Check sheet for the modelled part. Datum: model origin and axes. Units: mm. Coordinates: 2 decimals unless noted, no trailing zeros. Write each loop counter-clockwise with the first axis right and the second up, starting at its lowest first coordinate (ties: lowest second). Pieces come first, ordered by that corner, then holes. Notation, with made-up numbers: (-26, -12) -> (13, -12) arc R21 ccw to (13, 26) -> close; hole circle Ø1 at (41.25, -20). An arc over 180 degrees is marked (long way). Put each result on its own line as item: value.
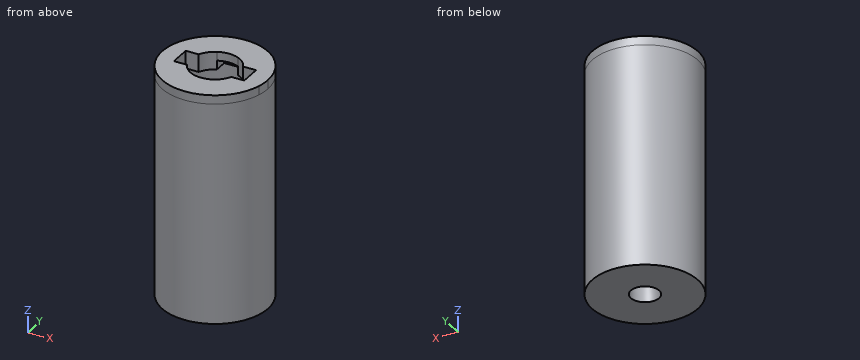
```python
from build123d import *
from build123d import SkipClean  # not in build123d's __all__

# Parameters (mm, degrees)
F1_DEPTH  = 2.5
F3_DEPTH  = 2.5
F6_ANGLE  = 90
F8_R      = 12.5
F9_DEPTH  = 2.5
F10_DEPTH = 2.5
F13_DEPTH = 2.5


with BuildPart() as f1:
    # F0 (on Front) → F1 (new body)
    with BuildSketch(Plane.XZ):
        with BuildLine():
            ThreePointArc((-66.598045975, 33.1235192716), (-51.598045975, 18.1235192716), (-36.598045975, 33.1235192716))
            ThreePointArc((-36.598045975, 33.1235192716), (-51.598045975, 48.1235192716), (-66.598045975, 33.1235192716))
        make_face()
        with BuildLine():
            ThreePointArc((-48.598045975, 39.4480745919), (-46.6482985067, 38.0732667399), (-45.2734906546, 36.1235192716))
            Line((-45.2734906546, 36.1235192716), (-41.598045975, 36.1235192716))
            Line((-41.598045975, 36.1235192716), (-41.598045975, 30.1235192716))
            Line((-41.598045975, 30.1235192716), (-45.2734906546, 30.1235192716))
            ThreePointArc((-45.2734906546, 30.1235192716), (-46.6482985067, 28.1737718033), (-48.598045975, 26.7989639513))
            Line((-48.598045975, 26.7989639513), (-48.598045975, 23.1235192716))
            Line((-48.598045975, 23.1235192716), (-54.598045975, 23.1235192716))
            Line((-54.598045975, 23.1235192716), (-54.598045975, 26.7989639513))
            ThreePointArc((-54.598045975, 26.7989639513), (-56.5477934433, 28.1737718033), (-57.9226012953, 30.1235192716))
            Line((-57.9226012953, 30.1235192716), (-61.598045975, 30.1235192716))
            Line((-61.598045975, 30.1235192716), (-61.598045975, 36.1235192716))
            Line((-61.598045975, 36.1235192716), (-57.9226012953, 36.1235192716))
            ThreePointArc((-57.9226012953, 36.1235192716), (-56.5477934433, 38.0732667399), (-54.598045975, 39.4480745919))
            Line((-54.598045975, 39.4480745919), (-54.598045975, 43.1235192716))
            Line((-54.598045975, 43.1235192716), (-48.598045975, 43.1235192716))
            Line((-48.598045975, 43.1235192716), (-48.598045975, 39.4480745919))
        make_face(mode=Mode.SUBTRACT)
    extrude(amount=F1_DEPTH)

    # F2 (on face) → F3 (join)
    with BuildSketch(Plane(origin=(0, 0, 0), x_dir=(-1, 0, 0), z_dir=(0, 1, 0))):
        with BuildLine():
            ThreePointArc((66.598045975, 33.1235192716), (66.0446186482, 37.1604163471), (64.4251742419, 40.899429535))
            ThreePointArc((64.4251742419, 40.899429535), (36.7710486733, 30.8519226932), (66.164820243, 29.5445407268))
            ThreePointArc((66.164820243, 29.5445407268), (66.4893456835, 31.3209674721), (66.598045975, 33.1235192716))
        make_face()
        with BuildLine():
            ThreePointArc((54.598045975, 39.4480745919), (56.5477934433, 38.0732667399), (57.9226012953, 36.1235192716))
            Line((57.9226012953, 36.1235192716), (61.598045975, 36.1235192716))
            Line((61.598045975, 36.1235192716), (61.598045975, 30.1235192716))
            Line((61.598045975, 30.1235192716), (57.9226012953, 30.1235192716))
            ThreePointArc((57.9226012953, 30.1235192716), (56.5477934433, 28.1737718033), (54.598045975, 26.7989639513))
            ThreePointArc((54.598045975, 26.7989639513), (51.598045975, 26.1235192716), (48.598045975, 26.7989639513))
            ThreePointArc((48.598045975, 26.7989639513), (46.6482985067, 28.1737718033), (45.2734906546, 30.1235192716))
            Line((45.2734906546, 30.1235192716), (41.598045975, 30.1235192716))
            Line((41.598045975, 30.1235192716), (41.598045975, 36.1235192716))
            Line((41.598045975, 36.1235192716), (45.2734906546, 36.1235192716))
            ThreePointArc((45.2734906546, 36.1235192716), (46.6482985067, 38.0732667399), (48.598045975, 39.4480745919))
            ThreePointArc((48.598045975, 39.4480745919), (51.598045975, 40.1235192716), (54.598045975, 39.4480745919))
        make_face(mode=Mode.SUBTRACT)
    with SkipClean():  # cleaning this boolean's faces spoils the solid; the shape is the same uncleaned
        extrude(amount=F3_DEPTH)


with BuildPart() as f5:
    # F4 (on Front) → F5 (revolve)
    with BuildSketch(Plane.XZ):
        Polygon((6.781338717, -22.533902707), (6.781338717, 37.466097293), (4.281338717, 37.466097293), (4.281338717, 7.466097293), (-3.218661283, 7.466097293), (-3.218661283, 2.466097293), (0.8746451318, -17.533902707), (-4.1253548682, -17.533902707), (-4.218661283, -22.533902707), align=None)
    revolve(axis=Axis((-8.218661283, 0, -12.1948756373), (0, 0, -1)))

    # F8 (on offset) → F9 (join)
    with BuildSketch(Plane.XY.offset(37.466097293)):
        with BuildLine():
            ThreePointArc((-23.218661283, 0), (-8.218661283, -15), (6.781338717, 0))
            ThreePointArc((6.781338717, 0), (-8.218661283, 15), (-23.218661283, 0))
        make_face()
        with Locations((-8.218661283, 0)):
            Circle(F8_R, mode=Mode.SUBTRACT)
    extrude(amount=F9_DEPTH)

    # F8 (on offset) → F10 (join)
    with BuildSketch(Plane.XY.offset(37.466097293)):
        with Locations((-8.218661283, 0)):
            Circle(F8_R)
        with BuildLine():
            ThreePointArc((-5.218661283, 6.3245553203), (-3.2689138147, 4.9497474683), (-1.8941059626, 3))
            Line((-1.8941059626, 3), (1.781338717, 3))
            Line((1.781338717, 3), (1.781338717, -3))
            Line((1.781338717, -3), (-1.8941059626, -3))
            ThreePointArc((-1.8941059626, -3), (-3.2689138147, -4.9497474683), (-5.218661283, -6.3245553203))
            Line((-5.218661283, -6.3245553203), (-5.218661283, -10))
            Line((-5.218661283, -10), (-11.218661283, -10))
            Line((-11.218661283, -10), (-11.218661283, -6.3245553203))
            ThreePointArc((-11.218661283, -6.3245553203), (-13.1684087513, -4.9497474683), (-14.5432166033, -3))
            Line((-14.5432166033, -3), (-18.218661283, -3))
            Line((-18.218661283, -3), (-18.218661283, 3))
            Line((-18.218661283, 3), (-14.5432166033, 3))
            ThreePointArc((-14.5432166033, 3), (-13.1684087513, 4.9497474683), (-11.218661283, 6.3245553203))
            Line((-11.218661283, 6.3245553203), (-11.218661283, 10))
            Line((-11.218661283, 10), (-5.218661283, 10))
            Line((-5.218661283, 10), (-5.218661283, 6.3245553203))
        make_face(mode=Mode.SUBTRACT)
    extrude(amount=F10_DEPTH)

    # F12 (on offset) → F13 (join)
    with BuildSketch(Plane.XY.offset(42.466097293)):
        with BuildLine():
            ThreePointArc((6.781338717, 0), (6.2279113902, 4.0368970755), (4.6084669839, 7.7759102634))
            ThreePointArc((4.6084669839, 7.7759102634), (-23.0456585847, -2.2715965784), (6.3481129851, -3.5789785448))
            ThreePointArc((6.3481129851, -3.5789785448), (6.6726384256, -1.8025517995), (6.781338717, 0))
        make_face()
        with BuildLine():
            ThreePointArc((-5.218661283, 6.3245553203), (-3.2689138147, 4.9497474683), (-1.8941059626, 3))
            Line((-1.8941059626, 3), (1.781338717, 3))
            Line((1.781338717, 3), (1.781338717, -3))
            Line((1.781338717, -3), (-1.8941059626, -3))
            ThreePointArc((-1.8941059626, -3), (-3.2689138147, -4.9497474683), (-5.218661283, -6.3245553203))
            ThreePointArc((-5.218661283, -6.3245553203), (-8.218661283, -7), (-11.218661283, -6.3245553203))
            ThreePointArc((-11.218661283, -6.3245553203), (-13.1684087513, -4.9497474683), (-14.5432166033, -3))
            Line((-14.5432166033, -3), (-18.218661283, -3))
            Line((-18.218661283, -3), (-18.218661283, 3))
            Line((-18.218661283, 3), (-14.5432166033, 3))
            ThreePointArc((-14.5432166033, 3), (-13.1684087513, 4.9497474683), (-11.218661283, 6.3245553203))
            ThreePointArc((-11.218661283, 6.3245553203), (-8.218661283, 7), (-5.218661283, 6.3245553203))
        make_face(mode=Mode.SUBTRACT)
    extrude(amount=-F13_DEPTH)


with BuildPart() as f1_1:
    # F6: moved
    add(f1.part.rotate(Axis((-43.4357683148, 2.5, 36.1235192716), (-1, 0, 0)), F6_ANGLE), clean=False)


solid = f5.part
```
Q1. Cross-section at C-C (z = -13). Record the cut outline in (x, y), plus the area to 3 significant figures.
Recorded:
outline: circle Ø30 at (-8.22, 0); hole circle Ø16.33 at (-8.22, 0)
area: 497 mm2
Q2. Depth check by flat-ended pin: P1, Ø1.2, axis at y = -7.5, z = 39.5, coming from the +X side; P2, Ø2.5, axis at y = 1.5, z = 39, coming from the -X side; P3, Ø6, axis at y = 9, z = -4.5, coming from the +X side. Enter the tip coordinate at first touch or a pass-through.
Recorded:
P1: stops at x = 5.1
P2: stops at x = -23.22
P3: stops at x = 5.53
Q3. Cross-section at B-B (x = 2.5). Record the cut outline in (y, z).
Recorded:
outline: (-10.49, -22.53) -> (10.49, -22.53) -> (10.49, 42.47) -> (-10.49, 42.47) -> close; hole (-6.43, 7.47) -> (6.43, 7.47) -> (6.43, 37.47) -> (-6.43, 37.47) -> close
Q4. Material ranges on line 1 along X through (y, z) = (0, 25.75); line 2 along X through (y, z) = (0, 4.95); line 3 along Z through (x, y) = (-2.75, 11), recorded low to high.
Recorded:
line 1: x = -23.22 to -20.72, 4.28 to 6.78
line 2: x = -23.22 to -13.22, -3.22 to 6.78
line 3: z = -22.53 to 7.47, 37.47 to 42.47
Q5. Cross-section at A-A (z = 27). Record the cut outline in (x, y), plus the area to 3 significant figures.
Recorded:
outline: circle Ø30 at (-8.22, 0); hole circle Ø25 at (-8.22, 0)
area: 216 mm2
